Source: CAD feature listing. Evaluate the final solid. Frame: model axes, mm. A direction names the side the tool comes from. Give positions to 0.01 mm unless a question says otherwise; leave off trailing zeros. Order: outer loops, then holes, each group sorted by start corner. A loop starts at its lowest first (then second) coordinate and runs counter-clockwise, first axis right, second up.
from build123d import *

# Parameters (mm, degrees)
BOSS_EXTRUDE1_START = 0.2
BOSS_EXTRUDE1_DEPTH = 12.4
SKETCH4_R           = 2.5
CUT_EXTRUDE1_DEPTH  = 12
SKETCH5_R           = 1.5
CUT_EXTRUDE2_DEPTH  = 12
BOSS_EXTRUDE3_DEPTH = 14.4
CIRPATTERN1_COUNT   = 2
CIRPATTERN1_ANGLE   = 90
CUT_EXTRUDE3_DEPTH  = 10
CHAMFER1_SIZE       = 2
FILLET1_R           = 2


with BuildPart() as part:
    # Sketch3 → Boss-Extrude1 (new body)
    with BuildSketch(Plane.ZY.offset(6.000000089).offset(BOSS_EXTRUDE1_START)):
        Polygon((5.2, 81), (5.2, 105.05), (-5.2, 105.05), (-5.2, 81), (-15.2, 81), (-15.2, 83), (-7.2, 83), (-7.2, 107.05), (7.2, 107.05), (7.2, 85.378651171), (7.2, 83), (15.2, 83), (15.2, 81), align=None)
    extrude(amount=-BOSS_EXTRUDE1_DEPTH)

    # Sketch4 → Cut-Extrude1 (cut)
    with BuildSketch(Plane(origin=(0, 107.05, 0), x_dir=(1, 0, 0), z_dir=(0, 1, 0))):
        with Locations(Location((0, 0, 0), (0, 0, 180))):
            Circle(SKETCH4_R)
    extrude(amount=-CUT_EXTRUDE1_DEPTH, mode=Mode.SUBTRACT)

    # Sketch5 → Cut-Extrude2 (cut)
    with BuildSketch(Plane(origin=(0, 83, 0), x_dir=(1, 0, 0), z_dir=(0, 1, 0))):
        with Locations(Location((-1.03e-07, 12, 0), (0, 0, 180))):
            Circle(SKETCH5_R)
        with Locations(Location((-1.03e-07, -12, 0), (0, 0, 180))):
            Circle(SKETCH5_R)
    cut_extrude2 = extrude(amount=-CUT_EXTRUDE2_DEPTH, mode=Mode.SUBTRACT)

    # Sketch7 → Boss-Extrude3 (add)
    with BuildSketch(Plane(origin=(0, 0, -7.2), x_dir=(-1, 0, 0), z_dir=(0, 0, -1))):
        Polygon((14.200000089, 83), (14.200000089, 81), (6.200000089, 81), (6.200000089, 107.05), (8.200000089, 107.05), (8.200000089, 83), align=None)
        Polygon((-8.200000089, 107.05), (-6.200000089, 107.05), (-6.200000089, 81), (-14.200000089, 81), (-14.200000089, 83), (-8.200000089, 83), align=None)
    extrude(amount=-BOSS_EXTRUDE3_DEPTH)

    # CirPattern1: Cut-Extrude2 ×2 about axis
    cirpattern1_axis = Axis((0, 0, 0), (0, 1, 0))
    for i in range(1, CIRPATTERN1_COUNT):
        add(cut_extrude2.rotate(cirpattern1_axis, i * CIRPATTERN1_ANGLE / (CIRPATTERN1_COUNT - 1)), mode=Mode.SUBTRACT)

    # Sketch11 → Cut-Extrude3 (cut)
    with BuildSketch(Plane(origin=(0, 83, 0), x_dir=(1, 0, 0), z_dir=(0, 1, 0))):
        with BuildLine():
            Line((18.453361638, 5.717898617), (11.935828042, 9.084933074))
            ThreePointArc((11.935828042, 9.084933074), (10.606601718, 10.606601718), (9.084933074, 11.935828042))
            Line((9.084933074, 11.935828042), (5.717898617, 18.453361638))
            Line((5.717898617, 18.453361638), (-5.717898617, 18.453361638))
            Line((-5.717898617, 18.453361638), (-9.084933074, 11.935828042))
            ThreePointArc((-9.084933074, 11.935828042), (-10.606601718, 10.606601718), (-11.935828042, 9.084933074))
            Line((-11.935828042, 9.084933074), (-18.453361638, 5.717898617))
            Line((-18.453361638, 5.717898617), (-18.453361638, -5.717898617))
            Line((-18.453361638, -5.717898617), (-11.935828042, -9.084933074))
            ThreePointArc((-11.935828042, -9.084933074), (-10.606601718, -10.606601718), (-9.084933074, -11.935828042))
            Line((-9.084933074, -11.935828042), (-5.717898617, -18.453361638))
            Line((-5.717898617, -18.453361638), (5.717898617, -18.453361638))
            Line((5.717898617, -18.453361638), (9.084933074, -11.935828042))
            ThreePointArc((9.084933074, -11.935828042), (10.606601718, -10.606601718), (11.935828042, -9.084933074))
            Line((11.935828042, -9.084933074), (18.453361638, -5.717898617))
            Line((18.453361638, -5.717898617), (18.453361638, 5.717898617))
        make_face()
        with BuildLine():
            Line((16.453361638, 4.5), (10.602285857, 7.522734517))
            ThreePointArc((10.602285857, 7.522734517), (9.192388155, 9.192388155), (7.522734517, 10.602285857))
            Line((7.522734517, 10.602285857), (4.5, 16.453361638))
            Line((4.5, 16.453361638), (-4.5, 16.453361638))
            Line((-4.5, 16.453361638), (-7.522734517, 10.602285857))
            ThreePointArc((-7.522734517, 10.602285857), (-9.192388155, 9.192388155), (-10.602285857, 7.522734517))
            Line((-10.602285857, 7.522734517), (-16.453361638, 4.5))
            Line((-16.453361638, 4.5), (-16.453361638, -4.5))
            Line((-16.453361638, -4.5), (-10.602285857, -7.522734517))
            ThreePointArc((-10.602285857, -7.522734517), (-9.192388155, -9.192388155), (-7.522734517, -10.602285857))
            Line((-7.522734517, -10.602285857), (-4.5, -16.453361638))
            Line((-4.5, -16.453361638), (4.5, -16.453361638))
            Line((4.5, -16.453361638), (7.522734517, -10.602285857))
            ThreePointArc((7.522734517, -10.602285857), (9.192388155, -9.192388155), (10.602285857, -7.522734517))
            Line((10.602285857, -7.522734517), (16.453361638, -4.5))
            Line((16.453361638, -4.5), (16.453361638, 4.5))
        make_face(mode=Mode.SUBTRACT)
    extrude(amount=-CUT_EXTRUDE3_DEPTH, mode=Mode.SUBTRACT)

    # Chamfer1
    chamfer1_edges = [part.edges().sort_by_distance(p)[0] for p in [
        (-6.200000089, 82, 7.2),
        (6.200000089, 82, -7.2),
        (6.200000089, 82, 7.2),
    ]]
    chamfer(chamfer1_edges, length=CHAMFER1_SIZE)

    # Fillet1
    # the kernel refuses this fillet: 2 mm, written as the material it takes off along each edge
    with BuildSketch(Plane(origin=(-6.200000089, 105.05, -5.2), x_dir=(0, 1, 0), z_dir=(0, 0, -1))) as fillet1_piece_1_section:
        Polygon((0, 0), (FILLET1_R * 1.02, 0), (FILLET1_R * 1.02, -FILLET1_R * 1.02), (0, -FILLET1_R * 1.02), align=None)
    fillet1_piece_1 = extrude(amount=FILLET1_R * 1.02, mode=Mode.PRIVATE)
    fillet1_piece_1 = fillet1_piece_1 - Plane(origin=(-6.200000089, 105.05, -5.2), x_dir=(0.7071067811865474, -0.7071067811865478, 5.985977498731896e-15), z_dir=(0, 0, -1)) * Sphere(FILLET1_R, mode=Mode.PRIVATE)
    add(fillet1_piece_1, mode=Mode.SUBTRACT)
    with BuildSketch(Plane(origin=(6.200000089, 105.05, -5.2), x_dir=(0, 0, -1), z_dir=(1, 0, 0))) as fillet1_piece_2_section:
        Polygon((0, 0), (FILLET1_R * 1.02, 0), (FILLET1_R * 1.02, FILLET1_R * 1.02), (0, FILLET1_R * 1.02), align=None)
    fillet1_piece_2 = extrude(amount=FILLET1_R * 1.02, mode=Mode.PRIVATE)
    fillet1_piece_2 = fillet1_piece_2 - Plane(origin=(6.200000089, 105.05, -5.2), x_dir=(-6.4472925120618815e-15, -0.7071067811865475, 0.7071067811865475), z_dir=(1, 0, 0)) * Sphere(FILLET1_R, mode=Mode.PRIVATE)
    add(fillet1_piece_2, mode=Mode.SUBTRACT)
    with BuildSketch(Plane(origin=(6.200000089, 105.05, 5.2), x_dir=(0, 0, 1), z_dir=(1, 0, 0))) as fillet1_piece_3_section:
        Polygon((0, 0), (FILLET1_R * 1.02, 0), (FILLET1_R * 1.02, -FILLET1_R * 1.02), (0, -FILLET1_R * 1.02), align=None)
    fillet1_piece_3 = extrude(amount=FILLET1_R * 1.02, mode=Mode.PRIVATE)
    fillet1_piece_3 = fillet1_piece_3 - Plane(origin=(6.200000089, 105.05, 5.2), x_dir=(5.5246624854019046e-15, -0.7071067811865475, -0.7071067811865475), z_dir=(1, 0, 0)) * Sphere(FILLET1_R, mode=Mode.PRIVATE)
    add(fillet1_piece_3, mode=Mode.SUBTRACT)
    with BuildSketch(Plane(origin=(-6.200000089, 105.05, 5.2), x_dir=(0, 1, 0), z_dir=(0, 0, 1))) as fillet1_piece_4_section:
        Polygon((0, 0), (FILLET1_R * 1.02, 0), (FILLET1_R * 1.02, FILLET1_R * 1.02), (0, FILLET1_R * 1.02), align=None)
    fillet1_piece_4 = extrude(amount=FILLET1_R * 1.02, mode=Mode.PRIVATE)
    fillet1_piece_4 = fillet1_piece_4 - Plane(origin=(-6.200000089, 105.05, 5.2), x_dir=(0.7071067811865474, -0.7071067811865478, 5.985977498731896e-15), z_dir=(0, 0, 1)) * Sphere(FILLET1_R, mode=Mode.PRIVATE)
    add(fillet1_piece_4, mode=Mode.SUBTRACT)
    with BuildSketch(Plane(origin=(-6.200000089, 107.05, -7.2), x_dir=(0, 0, 1), z_dir=(1, 0, 0)), Plane(origin=(6.200000089, 107.05, 7.2), x_dir=(0, 0, -1), z_dir=(-1, 0, 0))) as fillet1_piece_5:
        with BuildLine():
            CenterArc((FILLET1_R, FILLET1_R), FILLET1_R, 180, 90)
            Line((0, FILLET1_R), (0, 0))
            Line((0, 0), (FILLET1_R, 0))
        make_face()
    extrude(amount=12.400000179, mode=Mode.SUBTRACT)
    with BuildSketch(Plane(origin=(-8.200000089, 105.05, -7.2), x_dir=(0, 0, 1), z_dir=(0, -1, 0)), Plane(origin=(8.200000089, 83, -7.2), x_dir=(0, 0, 1), z_dir=(0, 1, 0))) as fillet1_piece_6:
        with BuildLine():
            CenterArc((FILLET1_R, -FILLET1_R), FILLET1_R, 90, 90)
            Line((0, -FILLET1_R), (0, 0))
            Line((0, 0), (FILLET1_R, 0))
        make_face()
    extrude(amount=22.05, mode=Mode.SUBTRACT)
    with BuildSketch(Plane(origin=(-8.200000089, 105.05, 7.2), x_dir=(0, 0, -1), z_dir=(0, -1, 0)), Plane(origin=(8.200000089, 83, 7.2), x_dir=(0, 0, -1), z_dir=(0, 1, 0))) as fillet1_piece_7:
        with BuildLine():
            CenterArc((FILLET1_R, FILLET1_R), FILLET1_R, 180, 90)
            Line((0, FILLET1_R), (0, 0))
            Line((0, 0), (FILLET1_R, 0))
        make_face()
    extrude(amount=22.05, mode=Mode.SUBTRACT)
    with BuildSketch(Plane(origin=(-8.200000089, 107.05, -5.2), x_dir=(1, 0, 0), z_dir=(0, 0, 1))) as fillet1_piece_8:
        with BuildLine():
            CenterArc((FILLET1_R, -FILLET1_R), FILLET1_R, 90, 90)
            Line((0, -FILLET1_R), (0, 0))
            Line((0, 0), (FILLET1_R, 0))
        make_face()
    extrude(amount=10.4, mode=Mode.SUBTRACT)
    with BuildSketch(Plane(origin=(8.200000089, 107.05, -5.2), x_dir=(-1, 0, 0), z_dir=(0, 0, 1))) as fillet1_piece_9:
        with BuildLine():
            CenterArc((FILLET1_R, FILLET1_R), FILLET1_R, 180, 90)
            Line((0, FILLET1_R), (0, 0))
            Line((0, 0), (FILLET1_R, 0))
        make_face()
    extrude(amount=10.4, mode=Mode.SUBTRACT)


solid = part.part
1) Ray query, L1, parallel to Z at x = 0, y = 81.7; L2, parallel to X at y = 82.3, z = 0; L3, parallel to Z at x = 0, y = 91.5. Return the intervals inside material, ascending.
Checks:
L1: z = -15.2 to -13.5, -10.5 to -5.2, 5.2 to 10.5, 13.5 to 15.2
L2: x = -14.2 to -13.5, -10.5 to -6.2, 6.2 to 10.5, 13.5 to 14.2
L3: z = -7.2 to -5.2, 5.2 to 7.2
2) Section query B-B on z = 12. Output: boundary loops of the cut face in (x, y).
Checks:
outline: (-6.2, 81) - (-1.5, 81) - (-1.5, 83) - (-6.2, 83) - close; (1.5, 81) - (6.2, 81) - (6.2, 83) - (1.5, 83) - close
3) Section query C-C on x = 1. Output: boundary loops of the cut face in (y, z), and give its area (3 significant figures).
Checks:
outline: (81, -15.2) - (83, -15.2) - (83, -13.12) - (81, -13.12) - close; (81, -10.88) - (83, -10.88) - (83, -7.2) - (105.05, -7.2) arc R2 ccw to (107.05, -5.2) - (107.05, -2.29) - (105.05, -2.29) - (105.05, -5.2) - (81, -5.2) - close; (81, 5.2) - (105.05, 5.2) - (105.05, 2.29) - (107.05, 2.29) - (107.05, 5.2) arc R2 ccw to (105.05, 7.2) - (83, 7.2) - (83, 10.88) - (81, 10.88) - close; (81, 13.12) - (83, 13.12) - (83, 15.2) - (81, 15.2) - close
area: 137 mm2
4) Pull-direction query (X, two-part tool) for faces 1 (the face through (-14.2, 82, 0)), 2 (the face through (2.5, 106.1, 0.1)), 3 (the face through (12.734, 82.014, -6.421)); classes: +X half, -X half, draft (parallel to the pull), parting line (faces both ways), or undercut.
Checks:
face 1: -X half
face 2: undercut
face 3: +X half
5) Reachability of faces 4 (the face through (-6.2, 82, -10)), 5 (the face through (-8.2, 94, 0)), 6 (the face through (6.2, 93, 0)) from +Z, -Z, +X, -X, +Y, -Y: full face, straight path, thin tool, end or side. Return the list, or none.
Checks:
face 4: -Z, -X, +Y, -Y
face 5: +Z, -Z, -X, +Y
face 6: -Y
6) Section query D-D on x = 12. Output: boundary loops of the cut face in (y, z).
Checks:
outline: (81, -6.8) - (83, -6.8) - (83, -1.5) - (81, -1.5) - close; (81, 1.5) - (83, 1.5) - (83, 6.8) - (81, 6.8) - close
7) First-contact query: pin 1 Ø6 at (x, y) = (4.5, 101) entering from -Z; pin 2 Ø3.5 at (x, y) = (-2.5, 96.5) entering from +Z; pin 3 Ø2 at (x, y) = (9, 82) entering from +Z; pin 4 Ø1.8 at (x, z) = (0, 12) entering from -Y. Flat tips, straight axial feed; report the tip coordinate or a pass-through.
Checks:
pin 1: stops at z = -7.2
pin 2: stops at z = 7.2
pin 3: stops at z = 7.4
pin 4: passes through
8) Section query A-A on y = 89.5. Output: boundary loops of the cut face in (x, z), and give its area (3 significant figures).
Checks:
outline: (-8.2, -5.2) arc R2 ccw to (-6.2, -7.2) - (6.2, -7.2) arc R2 ccw to (8.2, -5.2) - (8.2, 5.2) arc R2 ccw to (6.2, 7.2) - (-6.2, 7.2) arc R2 ccw to (-8.2, 5.2) - close; hole (-6.2, -5.2) - (6.2, -5.2) - (6.2, 5.2) - (-6.2, 5.2) - close
area: 104 mm2
